Can you work these out from the model? Positions are in its coordinate system, mm. A direction names the side the tool comes from. Coordinates: 2 decimals unless noted, no trailing zeros. Order: outer loops, then holes, each group sorted by start corner. A loop starts at its lowest first (then second) coordinate and runs counter-clockwise, first axis right, second up. Notation, with made-up numbers: (64, 3.25) -> (90, 3.25) arc R18 ccw to (90, 29.25) -> close; hole circle Ø2 at (79, 78.5). An arc over 180 degrees is marked (long way). Return JSON: item names as keys, results as strings. Group by question number.
1) For pin 1 (22.5 mm diameter, centred on y = -4.5, z = 292, fed in from +X); pin 2 (3 mm diameter, centred on y = -12.5, z = 322, fed in from +X); pin 3 (22.5 mm diameter, centred on x = -1, z = 321.5, fed in from +Y), each with a flat end and sliding along its axis, tell me the tip position at first contact or that it passes through.
2) If I drill on probe 1 along Z at (x, y) = (-39, -5.5); probe 2 along Y at (x, z) = (-13.5, 242), over which ranges is the centre line in solid material (lowest first)? Write a range as from..to.
3) If we section it at A-A, the plane z = 290: Please give me the cut outline in (x, y).
4) For faces 1 (the flat face through (-19.05, 0, 296)), 2 (the cylindrical face through (17.55, -17.62, 295.8)), 3 (the flat face through (19.05, 0, 296)), which set-ups out of +Z, -Z, +X, -X, +Y, -Y let a thin tool reach every point of the face, with its end or its side?
5) If we section it at B-B, the plane x = 0: Please give me the cut outline in (y, z), then the cut area to 3 significant figures.
6) If we section it at D-D, the plane x = -23: Please give me the cut outline in (y, z), then the cut area to 3 significant figures.
from build123d import *

# Parameters (mm, degrees)
F0_W     = 49.6
F0_H     = 10
F3_DEPTH = 116.232
F4_R     = 5


with BuildPart() as f1:
    # F0 (on Front) → F1 (revolve)
    with BuildSketch(Plane.XZ):
        with Locations((24.8, 235.9674370289)):
            Rectangle(F0_W, F0_H)
    revolve(axis=Axis((0, 0, 235.9674370289), (0, 0, 1)))

    # F2 (on face) → F3 (join)
    with BuildSketch(Plane.XY.offset(240.9674370289)):
        with BuildLine():
            ThreePointArc((19.05, 14.05), (17.5855339059, 17.5855339059), (14.05, 19.05))
            Line((14.05, 19.05), (-14.05, 19.05))
            ThreePointArc((-14.05, 19.05), (-17.5855339059, 17.5855339059), (-19.05, 14.05))
            Line((-19.05, 14.05), (-19.05, -14.05))
            ThreePointArc((-19.05, -14.05), (-17.5855339059, -17.5855339059), (-14.05, -19.05))
            Line((-14.05, -19.05), (14.05, -19.05))
            ThreePointArc((14.05, -19.05), (17.5855339059, -17.5855339059), (19.05, -14.05))
            Line((19.05, -14.05), (19.05, 14.05))
        make_face()
    extrude(amount=F3_DEPTH)

    # F4
    f4_edges = [f1.edges().sort_by_distance(p)[0] for p in [
        (0, -19.05, 357.199437),
    ]]
    fillet(f4_edges, radius=F4_R)


solid = f1.part
Result sheet:
{
 "1": {"pin 1": "stops at x = 19.05", "pin 2": "stops at x = 19.05", "pin 3": "stops at y = 19.05"},
 "2": {"probe 1": "z = 230.97..240.97", "probe 2": "y = -19.05..19.05"},
 "3": {"outline": "(-19.05, -14.05) arc R5 ccw to (-14.05, -19.05) -> (14.05, -19.05) arc R5 ccw to (19.05, -14.05) -> (19.05, 14.05) arc R5 ccw to (14.05, 19.05) -> (-14.05, 19.05) arc R5 ccw to (-19.05, 14.05) -> close"},
 "4": {"face 1": "+Z, -X, +Y, -Y", "face 2": "+Z, +X, -Y", "face 3": "+Z, +X, +Y, -Y"},
 "5": {"outline": "(-49.6, 230.97) -> (49.6, 230.97) -> (49.6, 240.97) -> (19.05, 240.97) -> (19.05, 352.2) arc R5 ccw to (14.05, 357.2) -> (-14.05, 357.2) arc R5 ccw to (-19.05, 352.2) -> (-19.05, 240.97) -> (-49.6, 240.97) -> close", "area": "5,410 mm2"},
 "6": {"outline": "(-43.94, 230.97) -> (43.94, 230.97) -> (43.94, 240.97) -> (-43.94, 240.97) -> close", "area": "879 mm2"}
}
